For this review, take the finished solid that the model builds, in its own axes (mm). Give positions to 0.01 mm unless a question says otherwise; leave off trailing zeros. Write each loop counter-clockwise with the first axis right and the second up, starting at its lowest first coordinate (ties: lowest second). Pieces come first, ordered by that corner, then holes.
1) For P1, Ø5.5, axis at x = 0, y = 37.25, coming from the +Z side; P2, Ø5, axis at y = 27.5, z = 6.5, coming from the +X side; P3, Ø8, axis at x = 7, z = 8, coming from the -Y side; P4, Ø5, axis at x = -4, z = 13.5, coming from the +Y side (3 decimals), all flat-tipped, find the tip position at first contact; note any pin that passes through.
2) Wall thickness on line 1 along Y through (x, z) = (0, 7.75); line 2 along X through (y, z) = (27.5, 13.75); line 3 along Y through (x, z) = (-23.5, 6): over which ranges is each line inside the solid? List them lowest first.
3) We need section D-D on z = 9.5. Give the boundary of the cut face in (x, y).
4) We need section A-A on y = 0. Give the boundary of the cut face in (x, z).
5) We need section C-C on y = -37.25. Give the boundary of the cut face in (x, z), and give its area (3 significant figures).
from build123d import *

# Parameters (mm, degrees)
F0_R     = 45
F1_DEPTH = 15
F2_R     = 30
F3_DEPTH = 15.001
F4_R     = 4.5
F5_DEPTH = 15.001


with BuildPart() as f1:
    # F0 (on Top) → F1 (new body)
    with BuildSketch(Plane.XY):
        Circle(F0_R)
    extrude(amount=F1_DEPTH)

    # F2 (on face) → F3 (cut, through all)
    with BuildSketch(Plane.XY.offset(15)):
        Circle(F2_R)
    extrude(amount=-F3_DEPTH, mode=Mode.SUBTRACT)

    # F4 (on face) → F5 (cut, through all)
    with BuildSketch(Plane.XY.offset(15)):
        with Locations((0, 37.25)):
            Circle(F4_R)
        with Locations((-37.25, 0)):
            Circle(F4_R)
        with Locations((37.25, 0)):
            Circle(F4_R)
        with Locations((0, -37.25)):
            Circle(F4_R)
    extrude(amount=-F5_DEPTH, mode=Mode.SUBTRACT)


solid = f1.part
Results list:
1. P1: passes through
1. P2: stops at x = 37.42
1. P3: stops at y = -44.9
1. P4: stops at y = 44.975
2. line 1: y = -45 to -41.75, -32.75 to -30, 30 to 32.75, 41.75 to 45
2. line 2: x = -35.62 to -11.99, 11.99 to 35.62
2. line 3: y = -38.38 to -18.65, 18.65 to 38.38
3. outline: circle Ø90 at (0, 0); hole circle Ø9 at (-37.25, 0); hole circle Ø60 at (0, 0); hole circle Ø9 at (0, -37.25); hole circle Ø9 at (0, 37.25); hole circle Ø9 at (37.25, 0)
4. outline: (-45, 0) - (-41.75, 0) - (-41.75, 15) - (-45, 15) - close; (-32.75, 0) - (-30, 0) - (-30, 15) - (-32.75, 15) - close; (30, 0) - (32.75, 0) - (32.75, 15) - (30, 15) - close; (41.75, 0) - (45, 0) - (45, 15) - (41.75, 15) - close
5. outline: (-25.25, 0) - (-4.5, 0) - (-4.5, 15) - (-25.25, 15) - close; (4.5, 0) - (25.25, 0) - (25.25, 15) - (4.5, 15) - close
5. area: 622 mm2
